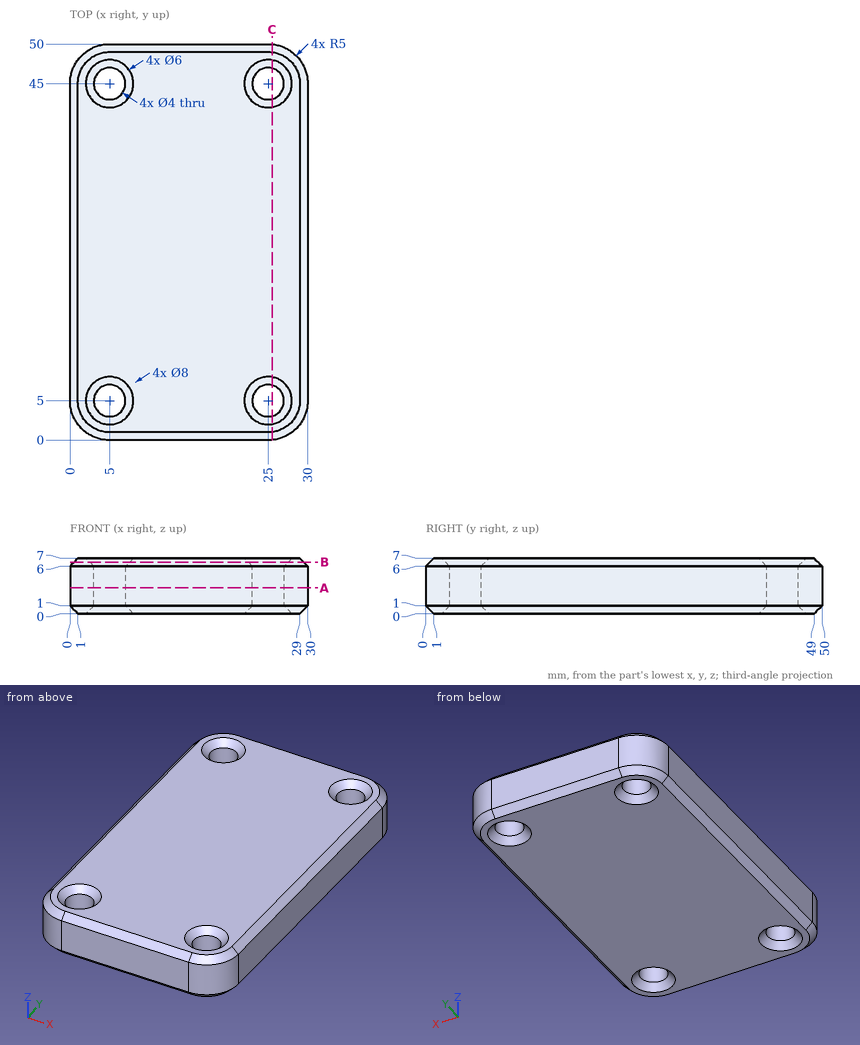
Geometry: see drawing. Coordinates: mm, zero at the bounding-box minimum. Coordinates: 2 decimals unless noted, no trailing zeros. Order: outer loops, then holes, each group sorted by start corner. A loop starts at its lowest first (then second) coordinate and runs counter-clockwise, first axis right, second up. Notation, with made-up numbers: (-35, -28) - (16, -28) arc R22 cw to (16, -14) - close; hole circle Ø2 at (65, 18.25). An arc over 180 degrees is marked (long way). Write each question's results on one line, items separated by ' | '.
1) Pin query (flat end, axial travel): pin 1 (5 mm diameter, centred on x = 25, y = 5, fed in from -Z); pin 2 (3 mm diameter, centred on x = 25, y = 45, fed in from -Z); pin 3 (4.5 mm diameter, centred on x = 5, y = 5, fed in from -Z). Return the tip coordinate at first contact, or that it passes through.
Results list:
pin 1: z = 0.5 | pin 2: through | pin 3: z = 0.75
2) Section C-C, the plane x = 25.5. State how many separate pieces and enclosed holes the cut face has, plus the area to 3 significant figures.
Results list:
separate pieces: 3 | enclosed holes: 0 | area: 289 mm^2
3) Line query: line 1 (Y direction, x = 5, z = 2.75); line 2 (X direction, y = 4.5, z = 1.25); line 3 (Z direction, x = 7.25, y = 3.5). Output: solid intervals per line, ascending. Write a range as from..to.
Results list:
line 1: 0..3, 7..43, 47..50 | line 2: 0.03..3.06, 6.94..23.06, 26.94..29.97 | line 3: 0.3..6.7
4) Section B-B, the plane z = 6.5. Return loops of the section in (x, y), plus the area to 3 significant figures.
Results list:
outline: (0.5, 5) arc R4.5 ccw to (5, 0.5) - (25, 0.5) arc R4.5 ccw to (29.5, 5) - (29.5, 45) arc R4.5 ccw to (25, 49.5) - (5, 49.5) arc R4.5 ccw to (0.5, 45) - close; hole circle Ø5 at (5, 5); hole circle Ø5 at (5, 45); hole circle Ø5 at (25, 5); hole circle Ø5 at (25, 45) | area: 1,330 mm^2
5) Section A-A, the plane z = 3.25. Return loops of the section in (x, y).
Results list:
outline: (0, 5) arc R5 ccw to (5, 0) - (25, 0) arc R5 ccw to (30, 5) - (30, 45) arc R5 ccw to (25, 50) - (5, 50) arc R5 ccw to (0, 45) - close; hole circle Ø4 at (5, 5); hole circle Ø4 at (5, 45); hole circle Ø4 at (25, 5); hole circle Ø4 at (25, 45)
